Drawing for the job (mm, zero at the part's lowest x, y, z). Give positions to 0.01 mm unless a question says otherwise; leave off trailing zeros. Loops run counter-clockwise (first coordinate to the right, second up) from the corner with the lowest first, then second, coordinate; pieces in that order, holes last. Notation, with made-up numbers: M 83.5,53 L 87.5,53 A27 ccw 87.5,82 Z; hole C 81.5,39 d1. An arc over 180 degrees is marked long. Answer in a Markdown table with one row per item. Add a question column.
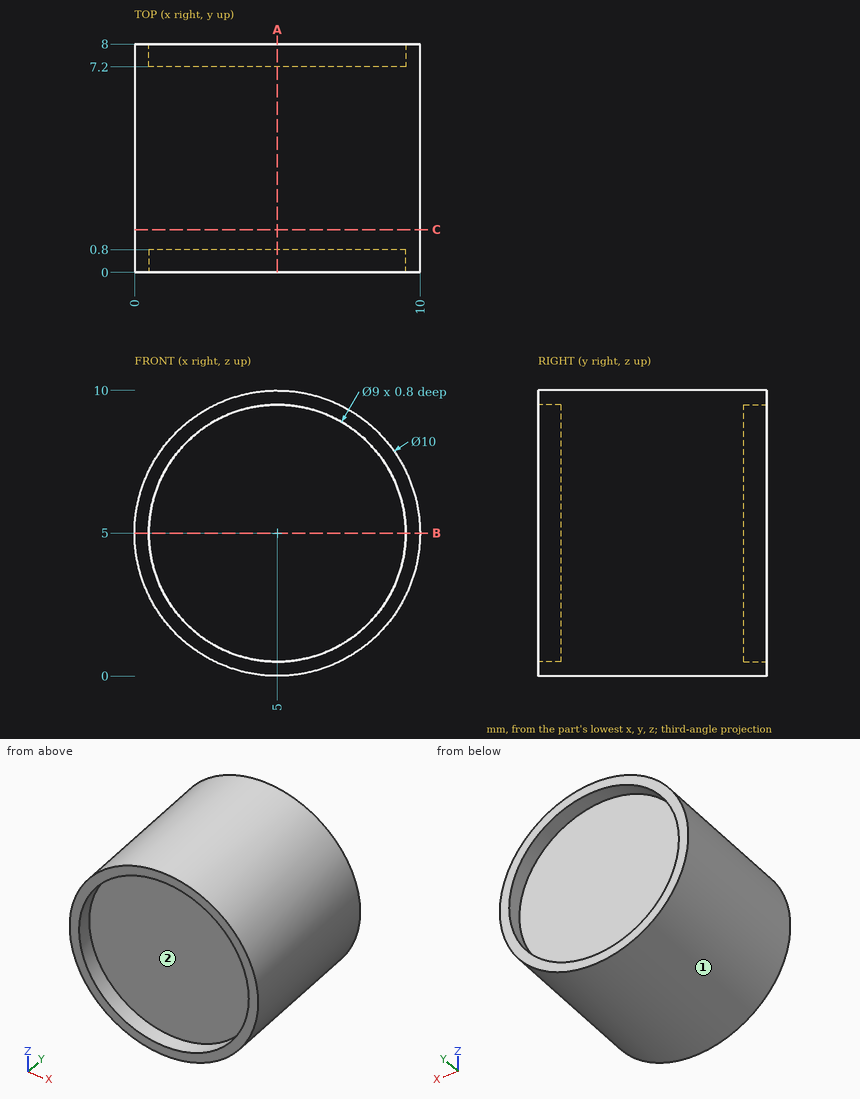
(1) Slice it at C-C, the plane y = 1.5. Give the cut face in (x, z), then the cut area to 3 significant figures.
(2) Slice it at A-A, the plane x = 5. Give the cut face in (y, z), then the cut area to 3 significant figures.
(3) Slice it at B-B, the plane z = 5. Give the cut face in (x, y).
(4) Wall check: line 1 (Z direction, x = 5, y = 0.2); line 2 (Y direction, x = 3.75, z = 9.25). Give the ranges that are in metal, low to high.
(5) Pull direction X, two halves, no side cores. Call the marked faces 1 and 2: +X half, -X half, draft (parallel to the pull), parting line (faces both ways), or undercut.
(6) Pin check, flat tips, straight feed: pin 1 (3 mm diameter, centred on y = 7, z = 2, fed in from -X); pin 2 (5.5 mm diameter, centred on x = 5, z = 5, fed in from -Y); pin 3 (1 mm diameter, centred on x = 6, z = 4, fed in from +Y). Stop position of each tip, or through.
Solution:
| question | item | result |
|---|---|---|
| 1 | outline | C 5,5 d10 |
| 1 | area | 78.5 mm^2 |
| 2 | outline | M 0,0 L 8,0 L 8,0.5 L 7.2,0.5 L 7.2,9.5 L 8,9.5 L 8,10 L 0,10 L 0,9.5 L 0.8,9.5 L 0.8,0.5 L 0,0.5 Z |
| 2 | area | 65.6 mm^2 |
| 3 | outline | M 0,0 L 0.5,0 L 0.5,0.8 L 9.5,0.8 L 9.5,0 L 10,0 L 10,8 L 9.5,8 L 9.5,7.2 L 0.5,7.2 L 0.5,8 L 0,8 Z |
| 4 | line 1 | 0 to 0.5, 9.5 to 10 |
| 4 | line 2 | 0.8 to 7.2 |
| 5 | face 1 | parting line |
| 5 | face 2 | undercut |
| 6 | pin 1 | x = 0.23 |
| 6 | pin 2 | y = 0.8 |
| 6 | pin 3 | y = 7.2 |
